Can you work these out from the model? Positions are in its coordinate system, mm. Face numbers are marked on the shaded views. A direction names the side the tool comes from. Coordinates: 2 decimals unless noted, no trailing zeros. Write each loop counter-clockwise with the first axis right and the second up, starting at its lowest first coordinate (ties: lowest second). Pieces come first, ordered by that corner, then holes. Notation, with made-up numbers: (66, 0.25) - (109, 0.25) arc R21 cw to (109, 36.25) - close; hole circle Ø7 at (77, 65). An arc over 180 degrees is marked (long way). Use one line per item in the form item = value. Start each with the question number.
(1) If we section it at C-C on x = 3.5: Please give me the cut outline in (y, z), then the cut area to 3 significant figures.
(2) If we section it at B-B on x = -10.25: Please give me the cut outline in (y, z), then the cut area to 3 significant figures.
(3) If we section it at A-A on z = -2.5: Please give me the cut outline in (x, y).
(4) Thinking about a two-plate mould opening in X: for the marked faces 4 and 5, which applies, pulls with the +X half, pulls with the -X half, needs draft (parallel to the pull), parting line crosses it, or undercut?
(5) For pin 1 Ø6.5 at (x, z) = (1, 1) entering from +Y; pin 2 Ø0.6 at (y, z) = (2, -5.5) entering from -X; pin 3 Ø0.6 at (x, y) = (-4, 2) entering from +Z, each with a flat end and sliding along its axis, tell me the tip position at first contact or that it passes through.
(6) If I drill on probe 1 along X at (y, z) = (0.4, -2.5); probe 2 along Y at (x, z) = (2.5, 5.25); probe 3 along X at (y, z) = (5.75, -6.25), over which ranges is the centre line in solid material (lowest first)? Write a range as from..to.
(7) On a 3-axis mill with a long thin cutter (end or side, diameter ignored), from which of +Z, -Z, +X, -X, +Y, -Y can I reach the whole of each face in a straight line? I mean the marked faces 1, 2 and 3. Say none if no direction works.
(8) If we section it at D-D on z = 8.25: Please give me the cut outline in (x, y), then the cut area to 3 significant figures.
```python
from build123d import *

# Parameters (mm, degrees)
SKETCH1_W           = 24
SKETCH1_H           = 21
SKETCH1_R           = 1.25
BOSS_EXTRUDE1_DEPTH = 1
SKETCH2_R           = 3
BOSS_EXTRUDE2_DEPTH = 6
SKETCH3_W           = 6.5
SKETCH3_H           = 6.5
SKETCH3_W_2         = 3.5
SKETCH3_H_2         = 10
BOSS_EXTRUDE3_DEPTH = 1.2


with BuildPart() as part:
    # Sketch1 → Boss-Extrude1 (new body)
    with BuildSketch(Plane(origin=(0, 0, 0), x_dir=(1, 0, 0), z_dir=(0, 1, 0))):
        Rectangle(SKETCH1_W, SKETCH1_H)
        with Locations(Location((-10.25, 2.5, 0), (0, 0, 270))):
            Circle(SKETCH1_R, mode=Mode.SUBTRACT)
    extrude(amount=BOSS_EXTRUDE1_DEPTH)

    # Sketch2 → Boss-Extrude2 (add)
    with BuildSketch(Plane(origin=(0, 1, 0), x_dir=(1, 0, 0), z_dir=(0, 1, 0))):
        with Locations(Location((3.5, 6.5, 0), (0, 0, 270))):
            Circle(SKETCH2_R)
        with Locations(Location((-3.5, 6.5, 0), (0, 0, 270))):
            Circle(SKETCH2_R)
    extrude(amount=BOSS_EXTRUDE2_DEPTH)

    # Sketch3 → Boss-Extrude3 (add)
    with BuildSketch(Plane(origin=(0, 1, 0), x_dir=(1, 0, 0), z_dir=(0, 1, 0))):
        with Locations((-3.5, 6.5)):
            Rectangle(SKETCH3_W, SKETCH3_H)
        with Locations((3.5, 6.5)):
            Rectangle(SKETCH3_W, SKETCH3_H)
        with Locations((0.25, -4.7)):
            Rectangle(SKETCH3_W_2, SKETCH3_H_2)
    extrude(amount=BOSS_EXTRUDE3_DEPTH)


solid = part.part
```
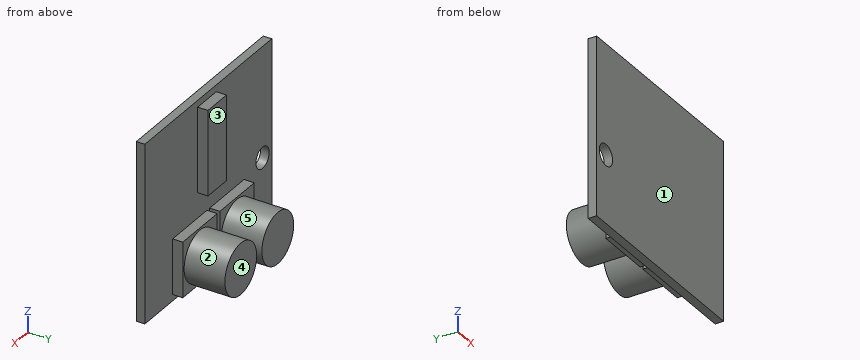
Reported:
q1.outline = (0, -10.5) - (1, -10.5) - (1, -9.75) - (2.2, -9.75) - (2.2, -9.5) - (7, -9.5) - (7, -3.5) - (2.2, -3.5) - (2.2, -3.25) - (1, -3.25) - (1, 10.5) - (0, 10.5) - close
q1.area = 57.6 mm2
q2.outline = (0, -10.5) - (1, -10.5) - (1, -3.75) - (0, -3.75) - close; (0, -1.25) - (1, -1.25) - (1, 10.5) - (0, 10.5) - close
q2.area = 18.5 mm2
q3.outline = (-12, 0) - (-11.5, 0) - (-11.5, 1) - (-12, 1) - close; (-9, 0) - (12, 0) - (12, 1) - (-9, 1) - close
q4.face_4 = needs draft
q4.face_5 = undercut
q5.pin_1 = 2.2
q5.pin_2 = -6.75
q5.pin_3 = -3.25
q6.probe_1 = -12..-11.5, -9..12
q6.probe_2 = 0..1
q6.probe_3 = -6.49..-0.51, 0.51..6.49
q7.face_1 = +Z, -Z, +X, -X, -Y
q7.face_2 = +Y
q7.face_3 = +Z, +X, -X, +Y
q8.outline = (-12, 0) - (12, 0) - (12, 1) - (2, 1) - (2, 2.2) - (-1.5, 2.2) - (-1.5, 1) - (-12, 1) - close
q8.area = 28.2 mm2
